Could you check a few things on this drawing? It's one solid part, dimensions in mm from its lowest x, y, z. A direction names the side the tool comes from. Coordinates: 2 decimals unless noted, no trailing zeros. Order: outer loops, then holes, each group sorted by start corner. A loop starts at its lowest first (then second) coordinate and runs counter-clockwise, first axis right, second up. Notation, with made-up numbers: (-38, 76.5) -> (13, 76.5) arc R25 cw to (13, 100.5) -> close; hole circle Ø5 at (81, 8). An arc over 180 degrees is marked (long way). Use a Markdown table: item, result. Add a question column.
1. If I drill on line 1 along Y through (x, z) = (6.5, 9.5); line 2 along X through (y, z) = (25, 5.5); line 3 along Z through (x, y) = (50.5, 30), over which ranges is the centre line in solid material (lowest first)? Write a range as from..to.
2. Suppose I cut it at A-A, the plane z = 8. List the corners of the cut face in (x, y) for me, then the cut area to 3 significant figures.
3. We'd pull the mould along Z, two halves only. Please class the marked faces 1, 2 and 3: pulls with the +Z half, pulls with the -Z half, needs draft (parallel to the pull), parting line crosses it, or undercut.
4. Suppose I cut it at D-D, the plane z = 24.5. List the corners of the cut face in (x, y) for me (1 decimal), then the cut area to 3 significant figures.
5. Suppose I cut it at C-C, the plane x = 12.5. List the corners of the cut face in (y, z) for me.
6. For the marked faces 4, 5 and 6, which set-ups out of +Z, -Z, +X, -X, +Y, -Y let a thin tool reach every point of the face, with its end or its side?
7. Suppose I cut it at B-B, the plane y = 24.5. List the corners of the cut face in (x, z) for me.
8. For pin 1 Ø3 at (x, z) = (14.5, 4) entering from +Y; pin 2 Ø10.5 at (x, y) = (50.5, 24) entering from +Z, each with a flat end and sliding along its axis, tell me the tip position at first contact or that it passes through.
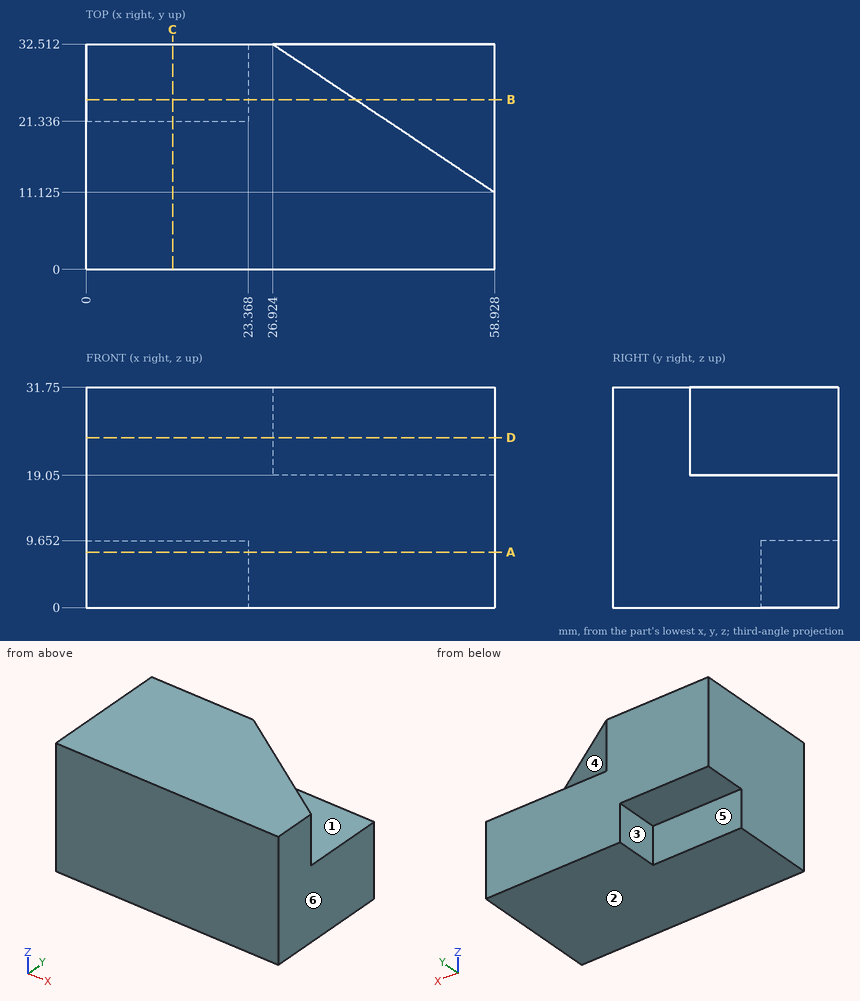
Worked out:
| question | item | result |
|---|---|---|
| 1 | line 1 | y = 0..21.34 |
| 1 | line 2 | x = 23.37..58.93 |
| 1 | line 3 | z = 0..19.05 |
| 2 | outline | (0, 0) -> (58.93, 0) -> (58.93, 32.51) -> (23.37, 32.51) -> (23.37, 21.34) -> (0, 21.34) -> close |
| 2 | area | 1,650 mm² |
| 3 | face 1 | pulls with the +Z half |
| 3 | face 2 | pulls with the -Z half |
| 3 | face 3 | needs draft |
| 4 | outline | (0, 0) -> (58.9, 0) -> (58.9, 11.1) -> (26.9, 32.5) -> (0, 32.5) -> close |
| 4 | area | 1,570 mm² |
| 5 | outline | (0, 0) -> (21.34, 0) -> (21.34, 9.65) -> (32.51, 9.65) -> (32.51, 31.75) -> (0, 31.75) -> close |
| 6 | face 4 | +Z, +X, +Y |
| 6 | face 5 | -Z, -X, +Y |
| 6 | face 6 | +Z, -Z, +X, +Y, -Y |
| 7 | outline | (0, 9.65) -> (23.37, 9.65) -> (23.37, 0) -> (58.93, 0) -> (58.93, 19.05) -> (38.91, 19.05) -> (38.91, 31.75) -> (0, 31.75) -> close |
| 8 | pin 1 | stops at y = 21.34 |
| 8 | pin 2 | stops at z = 19.05 |
